Can you work these out from the model? Positions are in its coordinate system, mm. Round coordinates to 2 decimals unless told otherwise and drop trailing zeros. Loops run counter-clockwise (first coordinate to the right, second up) from the corner with the lowest first, then second, coordinate; pieces in that order, holes last.
(1) Thinking about a two-plate mould opening in Z: for faces 1 (the face through (1, -1, 0)), 2 (the face through (1, -1, -20)), 3 (the face through (-0.487, -3.708, -10.056)), 4 (the face through (-0.59, -4.46, -17.41)), which applies, released by +Z, released by -Z, zero draft, split by the parting line, or undercut?
(2) I want a section at C-C on z = -8.25. Write out the boundary of the cut face in (x, y), plus the area to 3 significant figures.
(3) If I drill on line 1 along Y through (x, z) = (0, -10); line 2 along Z through (x, y) = (-2.25, 3.5); line 3 along Z through (x, y) = (-3.5, 1.5), over which ranges is the centre line in solid material (lowest first)?
(4) I want a section at D-D on z = -15. Write out the boundary of the cut face in (x, y).
(5) Will these pins go through, and if not, where does the flat tip stop? pin 1 Ø5 at (x, z) = (-3.5, -6) entering from -Y; pin 2 Ø5 at (x, z) = (0, -12) entering from +Y; pin 3 Ø4 at (x, z) = (0.5, -9.5) entering from +Y.
Autodesk Inventor part; units mm, degrees
ref_plane "YZ Plane" through (0, 0, 0) normal (1, 0, 0) x (0, 1, 0)
ref_plane "XZ Plane" through (0, 0, 0) normal (0, 1, 0) x (-1, 0, 0)
ref_plane "XY Plane" through (0, 0, 0) normal (0, 0, 1) x (1, 0, 0)
sketch "Sketch2" plane through (0, 0, 0) normal (0, 1, 0) x (-1, 0, 0)
  line L0 (0, 0) -> (-4.5, 0)
  line L1 (-4.5, 0) -> (-4.5, -6)
  line L2 (-4.5, -6) -> (0, -6)
  line L3 (0, -6) -> (0, 0)
  line L4 (0, -6) -> (-3.74, -6)
  line L5 (-3.74, -6) -> (-3.74, -14)
  line L6 (-3.74, -14) -> (0, -14)
  line L7 (0, -14) -> (0, -6)
  line L8 (0, -14) -> (-4.5, -14)
  line L9 (-4.5, -14) -> (-4.5, -20)
  line L10 (-4.5, -20) -> (0, -20)
  line L11 (0, -20) -> (0, -14)
  line L12 (0, 0) -> (-1, 0)
  line L13 (-1, 0) -> (-1, -20)
  line L14 (-1, -20) -> (0, -20)
  line L15 (0, -20) -> (0, 0)
  dimension "d0" = 1
  dimension "d1" = 6
  dimension "d2" = 4.5
  dimension "d3" = 20
  dimension "d4" = 6
  dimension "d6" = 4.5
revolve "Revolution1" add sketch "Sketch2" angle 360 about axis through (0, 0, -20) along (0, 0, 1)
revolve "Revolution2" cut sketch "Sketch2" angle 360 about axis through (0, 0, -6) along (0, 0, 1) contours L3 L2 L13 L0 | L7 L6 L13 L2 | L11 L10 L13 L6
chamfer "Chamfer1" distance 0.75 angle 45 2 edges at (-4.5, 0, -14) (-4.5, 0, -6)
equation "\"d4\" = d1"
equation "\"d6\" = d2"
properties part number "ShaftCoupler" material "Brass, Soft Yellow, Welded"
Filled sheet:
1. face 1: released by +Z
1. face 2: released by -Z
1. face 3: undercut
1. face 4: zero draft
2. outline: circle Ø7.48 at (0, 0); hole circle Ø2 at (0, 0)
2. area: 40.8 mm2
3. line 1: y = -3.74 to -1, 1 to 3.74
3. line 2: z = -20 to -14.41, -5.59 to 0
3. line 3: z = -20 to -14.06, -5.94 to 0
4. outline: circle Ø9 at (0, 0); hole circle Ø2 at (0, 0)
5. pin 1: stops at y = -4.36
5. pin 2: stops at y = 4.25
5. pin 3: stops at y = 3.74
